```python
from build123d import *

# Parameters (mm, degrees)
SKETCH_1_W          = 100
SKETCH_1_H          = 75
SKETCH_1_R          = 1.75
SKETCH_1_R_2        = 1.25
SKETCH_1_R_3        = 0.75
SKETCH_1_R_4        = 1.5
SKETCH_1_W_2        = 9
SKETCH_1_H_2        = 14.5
EXTRUDE_1_DEPTH     = 10
FILLET_5_R          = 6
CUT_EXTRUDE_1_REACH = 127.399
SKETCH_2_R          = 1.5
SKETCH_2_R_2        = 1.75
SKETCH_2_R_3        = 1
SKETCH_3_R          = 2.5
CUT_EXTRUDE_2_DEPTH = 7
SKETCH_4_W          = 2
SKETCH_4_H          = 2
EXTRUDE_2_DEPTH     = 2


with BuildPart() as part:
    # Эскиз1 → Бобышка-Вытянуть1 (new body)
    with BuildSketch(Plane(origin=(0, 0, 0), x_dir=(1, 0, 0), z_dir=(0, 1, 0))):
        with Locations((50, 37.5)):
            Rectangle(SKETCH_1_W, SKETCH_1_H)
        with Locations(Location((6, 69, 0), (0, 0, 270))):
            Circle(SKETCH_1_R, mode=Mode.SUBTRACT)
        with Locations(Location((94, 69, 0), (0, 0, 90))):
            Circle(SKETCH_1_R, mode=Mode.SUBTRACT)
        with Locations(Location((94, 6, 0), (0, 0, 270))):
            Circle(SKETCH_1_R, mode=Mode.SUBTRACT)
        with Locations(Location((6, 6, 0), (0, 0, 90))):
            Circle(SKETCH_1_R, mode=Mode.SUBTRACT)
        with Locations(Location((14, 68, 0), (0, 0, 270))):
            Circle(SKETCH_1_R_2, mode=Mode.SUBTRACT)
        with Locations(Location((32, 68, 0), (0, 0, 90))):
            Circle(SKETCH_1_R_2, mode=Mode.SUBTRACT)
        with Locations(Location((32, 7, 0), (0, 0, 270))):
            Circle(SKETCH_1_R_2, mode=Mode.SUBTRACT)
        with Locations(Location((14, 7, 0), (0, 0, 90))):
            Circle(SKETCH_1_R_2, mode=Mode.SUBTRACT)
        with Locations(Location((58.5, 65, 0), (0, 0, 270))):
            Circle(SKETCH_1_R_3, mode=Mode.SUBTRACT)
        with Locations(Location((77.5, 65, 0), (0, 0, 90))):
            Circle(SKETCH_1_R_3, mode=Mode.SUBTRACT)
        with Locations(Location((77.5, 10, 0), (0, 0, 270))):
            Circle(SKETCH_1_R_3, mode=Mode.SUBTRACT)
        with Locations(Location((58.5, 10, 0), (0, 0, 90))):
            Circle(SKETCH_1_R_3, mode=Mode.SUBTRACT)
        with Locations(Location((94, 37.5, 0), (0, 0, 270))):
            Circle(SKETCH_1_R_4, mode=Mode.SUBTRACT)
        with BuildLine():
            Line((16.5, 59), (29.5, 59))
            ThreePointArc((29.5, 59), (34.5, 54), (29.5, 49))
            Line((29.5, 49), (16.5, 49))
            ThreePointArc((16.5, 49), (11.5, 54), (16.5, 59))
        make_face(mode=Mode.SUBTRACT)
        with BuildLine():
            Line((16.5, 16), (29.5, 16))
            ThreePointArc((29.5, 16), (34.5, 21), (29.5, 26))
            Line((29.5, 26), (16.5, 26))
            ThreePointArc((16.5, 26), (11.5, 21), (16.5, 16))
        make_face(mode=Mode.SUBTRACT)
        with Locations((8, 37.5)):
            Rectangle(SKETCH_1_W_2, SKETCH_1_H_2, mode=Mode.SUBTRACT)
    extrude(amount=EXTRUDE_1_DEPTH)

    # Скругление5
    fillet_5_edges = [part.edges().sort_by_distance(p)[0] for p in [
        (0, 5, -75),
        (100, 5, -75),
        (100, 5, 0),
        (0, 5, 0),
    ]]
    fillet(fillet_5_edges, radius=FILLET_5_R)

    # Эскиз2 → Вырез-Вытянуть1 (cut, up to next)
    with BuildSketch(Plane.XZ, mode=Mode.PRIVATE) as cut_extrude_1_sk1:
        with Locations(Location((80, -7.5, 0), (0, 0, 270))):
            Circle(SKETCH_2_R)
    cut_extrude_1_tool1 = extrude(cut_extrude_1_sk1.sketch, amount=-CUT_EXTRUDE_1_REACH, mode=Mode.PRIVATE) & part.part
    # Эскиз2 → Вырез-Вытянуть1 (cut, up to next)
    with BuildSketch(Plane.XZ, mode=Mode.PRIVATE) as cut_extrude_1_sk2:
        with Locations(Location((50, -37.5, 0), (0, 0, 270))):
            Circle(SKETCH_2_R)
    cut_extrude_1_tool2 = extrude(cut_extrude_1_sk2.sketch, amount=-CUT_EXTRUDE_1_REACH, mode=Mode.PRIVATE) & part.part
    # Эскиз2 → Вырез-Вытянуть1 (cut, up to next)
    with BuildSketch(Plane.XZ, mode=Mode.PRIVATE) as cut_extrude_1_sk3:
        with Locations(Location((88, -62.75, 0), (0, 0, 270))):
            Circle(SKETCH_2_R_2)
    cut_extrude_1_tool3 = extrude(cut_extrude_1_sk3.sketch, amount=-CUT_EXTRUDE_1_REACH, mode=Mode.PRIVATE) & part.part
    # Эскиз2 → Вырез-Вытянуть1 (cut, up to next)
    with BuildSketch(Plane.XZ, mode=Mode.PRIVATE) as cut_extrude_1_sk4:
        with Locations(Location((88, -41.25, 0), (0, 0, 270))):
            Circle(SKETCH_2_R_2)
    cut_extrude_1_tool4 = extrude(cut_extrude_1_sk4.sketch, amount=-CUT_EXTRUDE_1_REACH, mode=Mode.PRIVATE) & part.part
    # Эскиз2 → Вырез-Вытянуть1 (cut, up to next)
    with BuildSketch(Plane.XZ, mode=Mode.PRIVATE) as cut_extrude_1_sk5:
        with Locations(Location((50, -22.5, 0), (0, 0, 270))):
            Circle(SKETCH_2_R)
    cut_extrude_1_tool5 = extrude(cut_extrude_1_sk5.sketch, amount=-CUT_EXTRUDE_1_REACH, mode=Mode.PRIVATE) & part.part
    # Эскиз2 → Вырез-Вытянуть1 (cut, up to next)
    with BuildSketch(Plane.XZ, mode=Mode.PRIVATE) as cut_extrude_1_sk6:
        with Locations(Location((65, -59, 0), (0, 0, 270))):
            Circle(SKETCH_2_R_3)
    cut_extrude_1_tool6 = extrude(cut_extrude_1_sk6.sketch, amount=-CUT_EXTRUDE_1_REACH, mode=Mode.PRIVATE) & part.part
    # Эскиз2 → Вырез-Вытянуть1 (cut, up to next)
    with BuildSketch(Plane.XZ, mode=Mode.PRIVATE) as cut_extrude_1_sk7:
        with Locations(Location((65, -45, 0), (0, 0, 270))):
            Circle(SKETCH_2_R_3)
    cut_extrude_1_tool7 = extrude(cut_extrude_1_sk7.sketch, amount=-CUT_EXTRUDE_1_REACH, mode=Mode.PRIVATE) & part.part
    add(cut_extrude_1_tool1.solids().sort_by_distance((80, 0, -7.5))[0], mode=Mode.SUBTRACT)
    add(cut_extrude_1_tool2.solids().sort_by_distance((50, 0, -37.5))[0], mode=Mode.SUBTRACT)
    add(cut_extrude_1_tool3.solids().sort_by_distance((88, 0, -62.75))[0], mode=Mode.SUBTRACT)
    add(cut_extrude_1_tool4.solids().sort_by_distance((88, 0, -41.25))[0], mode=Mode.SUBTRACT)
    add(cut_extrude_1_tool5.solids().sort_by_distance((50, 0, -22.5))[0], mode=Mode.SUBTRACT)
    add(cut_extrude_1_tool6.solids().sort_by_distance((65, 0, -59))[0], mode=Mode.SUBTRACT)
    add(cut_extrude_1_tool7.solids().sort_by_distance((65, 0, -45))[0], mode=Mode.SUBTRACT)

    # Эскиз3 → Вырез-Вытянуть2 (cut)
    with BuildSketch(Plane(origin=(0, 10, 0), x_dir=(1, 0, 0), z_dir=(0, 1, 0))):
        with Locations(Location((14, 68, 0), (0, 0, 270))):
            Circle(SKETCH_3_R)
        with Locations(Location((32, 68, 0), (0, 0, 270))):
            Circle(SKETCH_3_R)
        with Locations(Location((14, 7, 0), (0, 0, 270))):
            Circle(SKETCH_3_R)
        with Locations(Location((32, 7, 0), (0, 0, 270))):
            Circle(SKETCH_3_R)
    extrude(amount=-CUT_EXTRUDE_2_DEPTH, mode=Mode.SUBTRACT)

    # Эскиз4 → Бобышка-Вытянуть2 (add)
    with BuildSketch(Plane(origin=(0, 10, 0), x_dir=(1, 0, 0), z_dir=(0, 1, 0))):
        with Locations((94.855745834, 42)):
            Rectangle(SKETCH_4_W, SKETCH_4_H)
        with Locations((94.855745834, 62)):
            Rectangle(SKETCH_4_W, SKETCH_4_H)
    extrude(amount=EXTRUDE_2_DEPTH)


solid = part.part
```
Input: part model. Units: mm. Frame: model coordinates. A direction names the side the tool comes from. Coordinates: 2 decimals unless noted, no trailing zeros. Write each loop counter-clockwise with the first axis right and the second up, starting at its lowest first coordinate (ties: lowest second). Pieces come first, ordered by that corner, then holes. Notation, with made-up numbers: (13, 38.25) - (46, 38.25) arc R19 ccw to (46, 63.25) - close; hole circle Ø10 at (-17.75, -26.75). An arc over 180 degrees is marked (long way). Put each result on its own line as item: value. Start each with the question number.
1) Mould query, pull axis X, two halves, no side actions, for faces 4 (the face through (14.38, 1.48, -66.81)), 5 (the face through (49, 10, -46)), 6 (the face through (98.196, 5.07, -1.711)). Classes: pulls with the +X half, pulls with the -X half, needs draft (parallel to the pull), parting line crosses it, or undercut.
2) Cut plane D-D (x = 74.5). Return the cut outline in (y, z), plus the area to 3 significant figures.
3) Ray query, L1, parallel to Z at x = 77.5, y = 4.75; L2, parallel to X at y = 3.5, z = -10; L3, parallel to Z at x = 20.5, y = 1. Return the intervals inside material, ascending.
4) Cut plane C-C (y = 1.75). State how many separate pieces and enclosed holes the cut face has, plus the area to 3 significant figures.
5) Cut plane A-A (z = -54.5). Return the cut outline in (x, y), plus the area to 4 significant figures.
6) Cut plane B-B (x = 32). Return the cut outline in (y, z).
7) Contact query for flat-ended pins moving along their axis: pin 1 (0.6 mm diameter, centred on y = 11, z = -61.5, fed in from +X); pin 2 (3.5 mm diameter, centred on x = 94, z = -37.5, fed in from +Y); pin 3 (2 mm diameter, centred on y = 10.5, z = -39.5, fed in from -X); pin 4 (2 mm diameter, centred on y = 11.5, z = -42, fed in from -X). Output: stop coordinate, or through.
8) Reachability of faces 1 (the face through (93.856, 11, -42)), 2 (the face through (23, 5, -26)), 3 (the face through (12.5, 6.5, -70)) from +Z, -Z, +X, -X, +Y, -Y: full face, straight path, thin tool, end or side. Return the list, or none.
Resolved:
1. face 4: undercut
1. face 5: needs draft
1. face 6: pulls with the +X half
2. outline: (0, -75) - (10, -75) - (10, 0) - (0, 0) - close
2. area: 750 mm2
3. L1: z = -75 to -65.75, -64.25 to -10.75, -9.25 to 0
3. L2: x = 0 to 57.75, 59.25 to 76.75, 78.25 to 100
3. L3: z = -75 to -59, -49 to -26, -16 to 0
4. separate pieces: 1
4. enclosed holes: 23
4. area: 6,800 mm2
5. outline: (0, 0) - (11.53, 0) - (11.53, 10) - (0, 10) - close; (34.47, 0) - (100, 0) - (100, 10) - (34.47, 10) - close
5. area: 770.5 mm2
6. outline: (0, -75) - (10, -75) - (10, -70.5) - (3, -70.5) - (3, -69.25) - (0, -69.25) - close; (0, -66.75) - (3, -66.75) - (3, -65.5) - (10, -65.5) - (10, -58.33) - (0, -58.33) - close; (0, -49.67) - (10, -49.67) - (10, -25.33) - (0, -25.33) - close; (0, -16.67) - (10, -16.67) - (10, -9.5) - (3, -9.5) - (3, -8.25) - (0, -8.25) - close; (0, -5.75) - (3, -5.75) - (3, -4.5) - (10, -4.5) - (10, 0) - (0, 0) - close
7. pin 1: stops at x = 95.86
7. pin 2: stops at y = 10
7. pin 3: stops at x = 0
7. pin 4: stops at x = 93.86
8. face 1: +Z, -Z, -X, +Y
8. face 2: +Y, -Y
8. face 3: +Y
